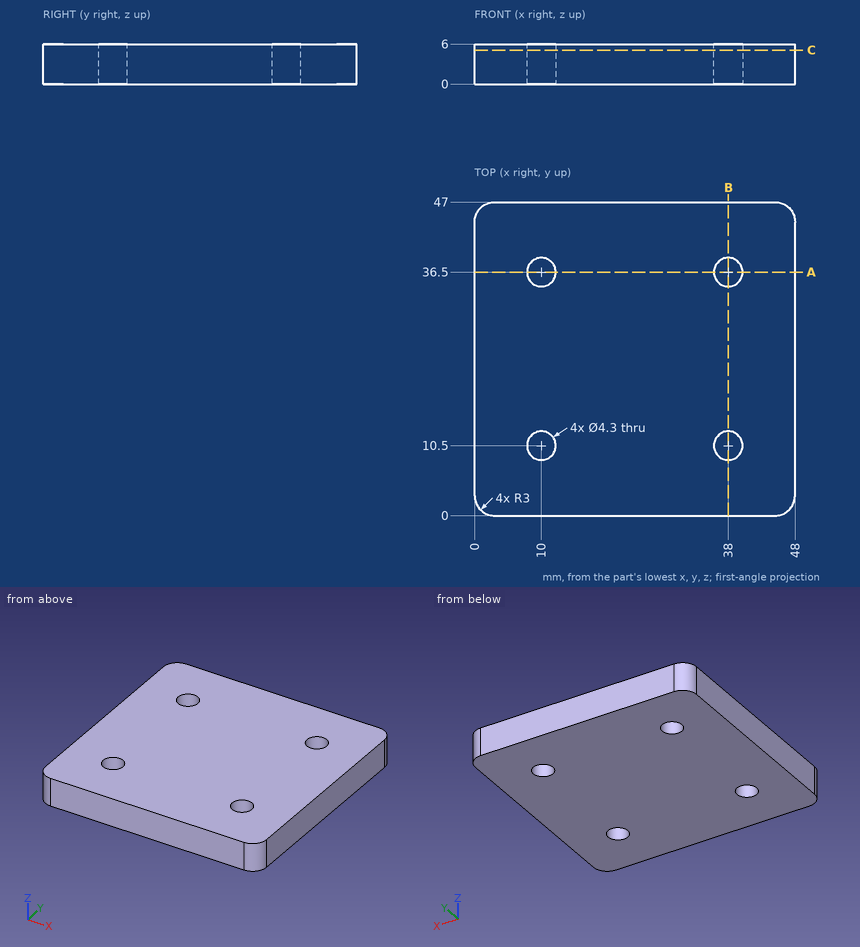
Input: dimensioned drawing with shaded views. Units: mm. Origin: part minimum x, y, z. Coordinates: 2 decimals unless noted, no trailing zeros. Write each loop counter-clockwise with the first axis right and the second up, starting at its lowest first coordinate (ties: lowest second). Pieces come first, ordered by that corner, then holes. Notation, with made-up numbers: M 62,-0.5 L 112,-0.5 A10 ccw 112,16.5 Z; hole C 24.25,-34 d1. An arc over 180 degrees is marked long. Answer as a JSON object with one key per item and string values. Group by question number.
(1) Section A-A on y = 36.5. Output: boundary loops of the cut face in (x, z), plus the area to 3 significant figures.
(2) Contact query for a flat-ended pin moving along its axis: P1, Ø4, axis at x = 38, y = 10.5, coming from the +Z side. Output: stop coordinate, or through.
(3) Ray query, line 1 along Y through (x, z) = (10, 4.85); line 2 along X through (y, z) = (9.5, 0.9); line 3 along Y through (x, z) = (37, 0.95). Return the intervals inside material, ascending. Write a range as [from, to].
(4) Section B-B on x = 38. Output: boundary loops of the cut face in (y, z).
(5) Section C-C on z = 5.1. Output: boundary loops of the cut face in (x, y), plus the area to 3 significant figures.
Result set:
{
 "1": {"outline": "M 0,0 L 7.85,0 L 7.85,6 L 0,6 Z; M 12.15,0 L 35.85,0 L 35.85,6 L 12.15,6 Z; M 40.15,0 L 48,0 L 48,6 L 40.15,6 Z", "area": "236 mm2"},
 "2": {"P1": "passes through"},
 "3": {"line 1": "y = [0, 8.35], [12.65, 34.35], [38.65, 47]", "line 2": "x = [0, 8.1], [11.9, 36.1], [39.9, 48]", "line 3": "y = [0, 8.6], [12.4, 34.6], [38.4, 47]"},
 "4": {"outline": "M 0,0 L 8.35,0 L 8.35,6 L 0,6 Z; M 12.65,0 L 34.35,0 L 34.35,6 L 12.65,6 Z; M 38.65,0 L 47,0 L 47,6 L 38.65,6 Z"},
 "5": {"outline": "M 0,3 A3 ccw 3,0 L 45,0 A3 ccw 48,3 L 48,44 A3 ccw 45,47 L 3,47 A3 ccw 0,44 Z; hole C 10,10.5 d4.3; hole C 10,36.5 d4.3; hole C 38,10.5 d4.3; hole C 38,36.5 d4.3", "area": "2,190 mm2"}
}
